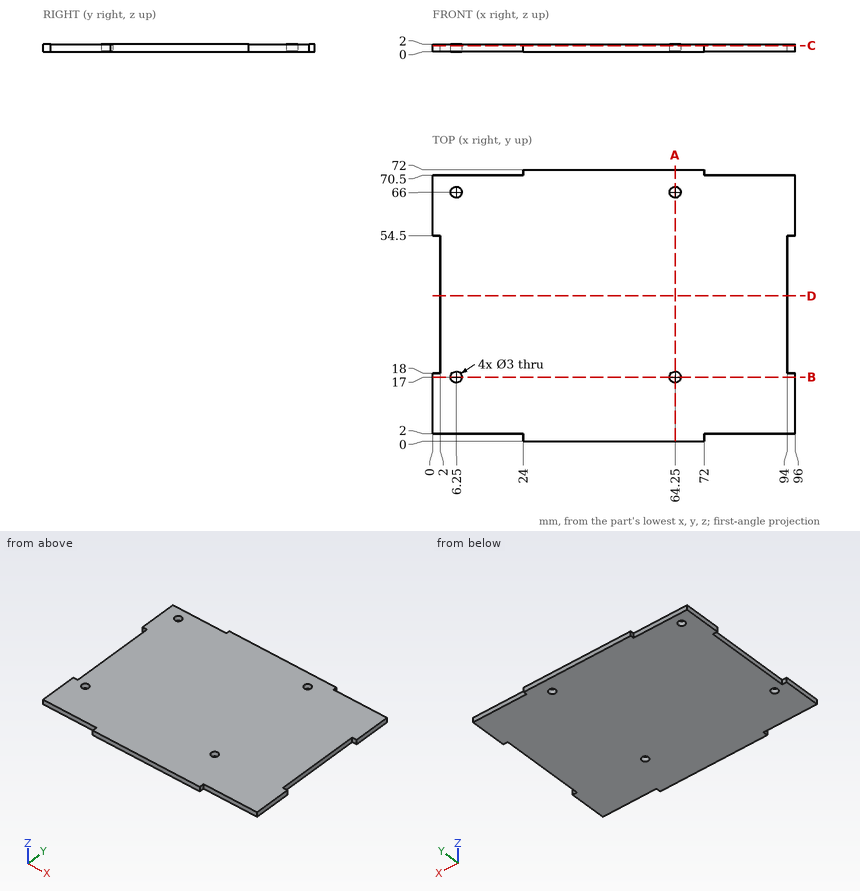
Design review of the part shown in the three views and the two pictorial views. Dimensions are in mm from the part's minimum x, y and z. Coordinates: 2 decimals unless noted, no trailing zeros. Write each loop counter-clockwise with the first axis right and the second up, starting at its lowest first coordinate (ties: lowest second). Pieces come first, ordered by that corner, then holes.
(1) Wall thickness on probe 1 along Y at (x, z) = (6.25, 1.65); probe 2 along X at (y, z) = (66, 0.85); probe 3 along Y at (x, z) = (5.5, 1.2): over which ranges is each line inside the solid? List them lowest first.
(2) Add section A-A on x = 64.25. Give the boundary of the cut face in (y, z), then the cut area to 3 significant figures.
(3) Add section C-C on z = 1.55. Give the boundary of the cut face in (x, y), then the cut area to 3 significant figures.
(4) Add section B-B on y = 17. Give the boundary of the cut face in (x, z).
(5) Add section D-D on y = 38.5. Give the boundary of the cut face in (x, z).
(6) For pin 1 Ø0.6 at (x, z) = (10.5, 1.5) entering from +Y; pin 2 Ø1.2 at (y, z) = (71.5, 1) entering from -X; pin 3 Ø4 at (x, y) = (64.25, 66) entering from +Z; pin 4 Ø1 at (y, z) = (1, 1) entering from +X, all flat-tipped, find the tip position at first contact; note any pin that passes through.
Answer sheet:
1. probe 1: y = 2 to 15.5, 18.5 to 64.5, 67.5 to 70.5
1. probe 2: x = 0 to 4.75, 7.75 to 62.75, 65.75 to 96
1. probe 3: y = 2 to 15.7, 18.3 to 64.7, 67.3 to 70.5
2. outline: (0, 0) - (15.5, 0) - (15.5, 2) - (0, 2) - close; (18.5, 0) - (64.5, 0) - (64.5, 2) - (18.5, 2) - close; (67.5, 0) - (72, 0) - (72, 2) - (67.5, 2) - close
2. area: 132 mm2
3. outline: (0, 2) - (24, 2) - (24, 0) - (72, 0) - (72, 2) - (96, 2) - (96, 18) - (94, 18) - (94, 54.5) - (96, 54.5) - (96, 70.5) - (72, 70.5) - (72, 72) - (24, 72) - (24, 70.5) - (0, 70.5) - (0, 54.5) - (2, 54.5) - (2, 18) - (0, 18) - close; hole circle Ø3 at (6.25, 17); hole circle Ø3 at (6.25, 66); hole circle Ø3 at (64.25, 17); hole circle Ø3 at (64.25, 66)
3. area: 6,570 mm2
4. outline: (0, 0) - (4.75, 0) - (4.75, 2) - (0, 2) - close; (7.75, 0) - (62.75, 0) - (62.75, 2) - (7.75, 2) - close; (65.75, 0) - (96, 0) - (96, 2) - (65.75, 2) - close
5. outline: (2, 0) - (94, 0) - (94, 2) - (2, 2) - close
6. pin 1: stops at y = 70.5
6. pin 2: stops at x = 24
6. pin 3: stops at z = 2
6. pin 4: stops at x = 72
